Study the drawing (mm; zero at the part's minimum x, y, z) and answer. A direction names the side the tool comes from. Coordinates: 2 decimals unless noted, no trailing zeros. Write each loop counter-clockwise with the first axis right and the second up, starting at its lowest first coordinate (ties: lowest second). Pieces come first, ordered by that corner, then holes. Notation, with made-up numbers: (-26.75, 55) -> (-5.75, 55) arc R26 ccw to (-5.75, 94) -> close; hole circle Ø4 at (5.5, 38). An arc over 180 degrees is marked (long way). Answer in a Markdown table with one row per item. Add a question column.
Item 1: Given pin 1 Ø13.5 at (y, z) = (36.5, 5.5) entering from +X; pin 2 Ø8.5 at (y, z) = (47.5, 12) entering from -X; pin 3 Ø4 at (x, y) = (59.5, 41.5) entering from +Z (3 decimals), each flat-ended and moving along its own axis, determine where each tip first touches the part or whether it passes through.
Item 2: Section C-C on z = 21.75 is taken. Write down the section's boundary in (x, y), then the cut area to 3 significant figures.
Item 3: Which of the six approach directions +Z, -Z, +X, -X, +Y, -Y give full straight-line access (tool end or side, diameter ignored) to the marked faces 1 and 2?
Item 4: Straight lines are drawn through the part: line 1 (Y direction, x = 216, z = 17.9); line 2 (X direction, y = 44.5, z = 3.75); line 3 (Z direction, x = 116.5, y = 26.5) (1 decimal). For each, find the intervals that lie inside material, in ascending order. Write a range as from..to.
Item 5: Section D-D on z = 6.25 is taken. Write down the section's boundary in (x, y), then the cut area to 3 significant figures.
Item 6: Section B-B on x = 14 is taken. Write down the section's boundary in (y, z) (1 decimal).
Item 7: Section A-A on y = 28 is taken. Write down the section's boundary in (x, z) (1 decimal).
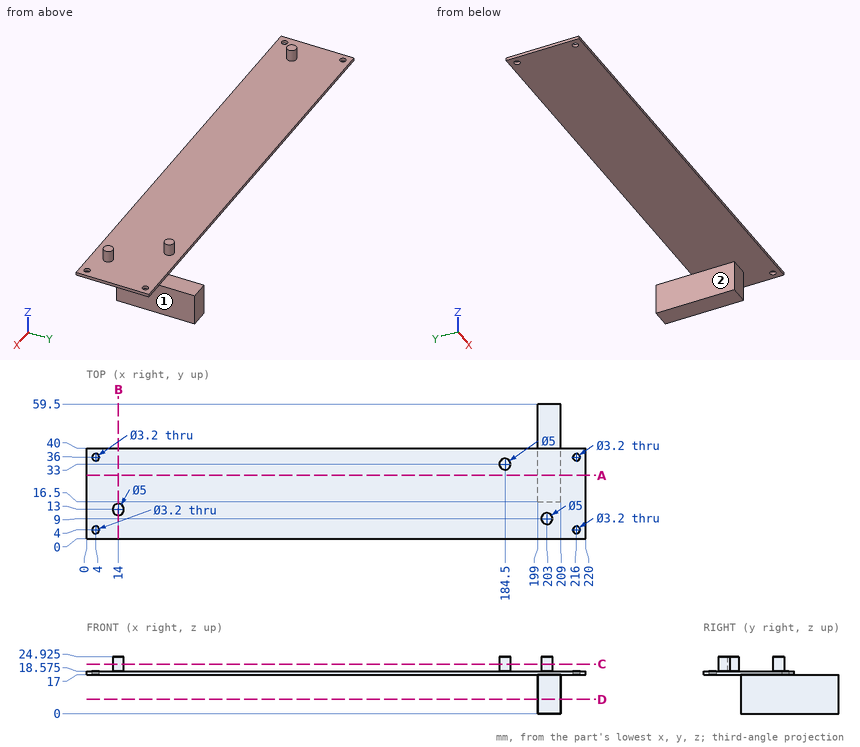
Results below:
| question | item | result |
|---|---|---|
| 1 | pin 1 | stops at x = 209 |
| 1 | pin 2 | stops at x = 199 |
| 1 | pin 3 | stops at z = 18.575 |
| 2 | outline | circle Ø5 at (14, 13); circle Ø5 at (184.5, 33); circle Ø5 at (203, 9) |
| 2 | area | 58.9 mm2 |
| 3 | face 1 | -Z, +X, +Y, -Y |
| 3 | face 2 | -Z, -X, +Y, -Y |
| 4 | line 1 | y = 0..2.4, 5.6..34.4, 37.6..40 |
| 4 | line 2 | x = 199..209 |
| 4 | line 3 | z = 17..18.6 |
| 5 | outline | (199, 16.5) -> (209, 16.5) -> (209, 59.5) -> (199, 59.5) -> close |
| 5 | area | 430 mm2 |
| 6 | outline | (0, 17) -> (40, 17) -> (40, 18.6) -> (15.5, 18.6) -> (15.5, 24.9) -> (10.5, 24.9) -> (10.5, 18.6) -> (0, 18.6) -> close |
| 7 | outline | (0, 17) -> (199, 17) -> (199, 0) -> (209, 0) -> (209, 17) -> (220, 17) -> (220, 18.6) -> (0, 18.6) -> close |
